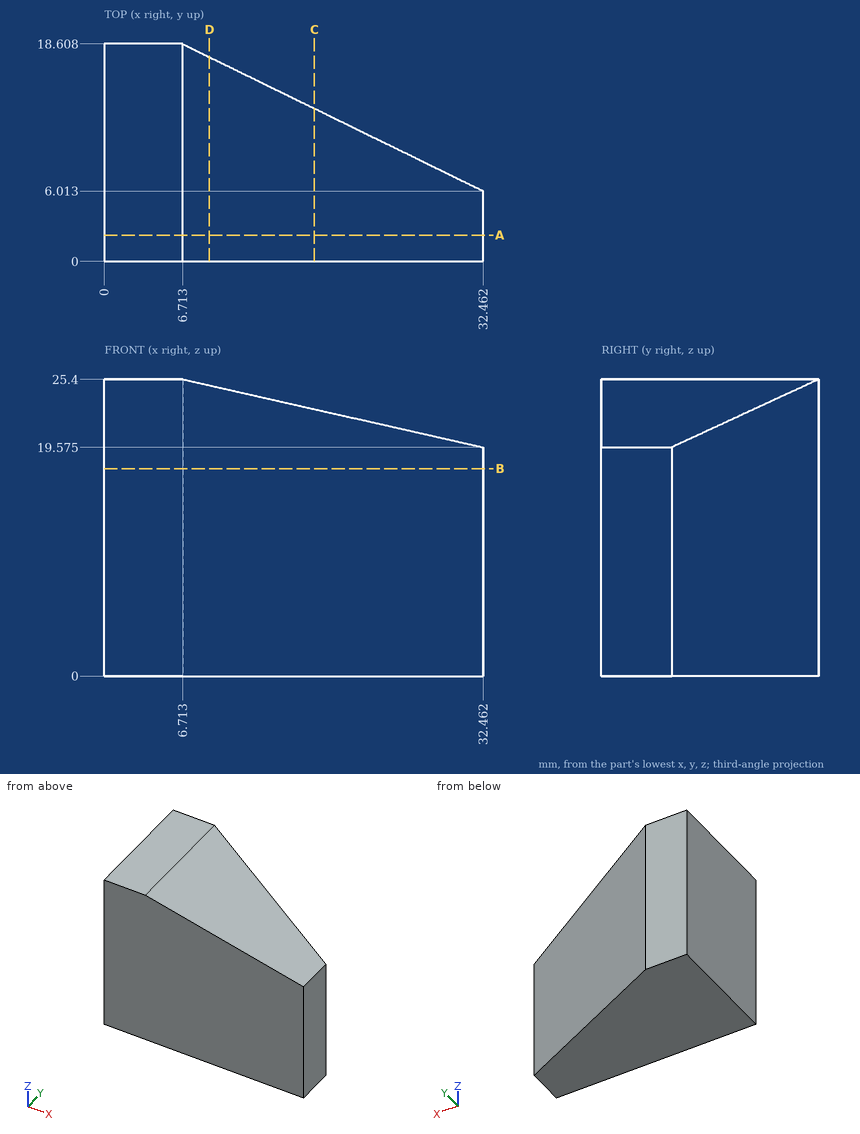
Verification items for this drawing (mm, ordinates from the low corner). Round coordinates to 2 decimals unless told otherwise and drop trailing zeros. Order: outer loops, then holes, each group sorted by start corner. A loop starts at its lowest first (then second) coordinate and runs counter-clockwise, first axis right, second up. Notation, with made-up numbers: (1.25, 64) - (16.25, 64) arc R19 cw to (16.25, 84) - close; hole circle Ø6 at (-34.5, -31.5). An arc over 180 degrees is marked (long way). Answer as CSV lines item,"result". Start each with the question number.
1) Section check D-D (x = 9). Record the cut outline in (y, z).
2) Scan lines: probe 1 along X at (y, z) = (14.25, 4.5) (1 decimal); probe 2 along Z at (x, y) = (24.5, 8.75) (1 decimal); probe 3 along Z at (x, y) = (15, 14.25) (1 decimal). Record each from-to range of solid material in increasing order.
3) Section check C-C (x = 18). Record the cut outline in (y, z).
4) Depth check by flat-ended pin: pin 1 (2 mm diameter, centred on x = 29, y = 11, fed in from +Z); pin 2 (6 mm diameter, centred on x = 25.5, z = 10, fed in from +Y) (1 decimal); pin 3 (5 mm diameter, centred on x = 27, z = 9.5, fed in from +Y). Enter the tip coordinate at first touch or a pass-through.
5) Section check A-A (y = 2.25). Record the cut outline in (x, z) (1 decimal).
6) Section check B-B (z = 17.75). Record the cut outline in (x, y).
Determined:
1,outline,"(0, 0) - (17.49, 0) - (17.49, 24.88) - (0, 24.88) - close"
2,probe 1,"0 to 15.6"
2,probe 2,"0 to 21.4"
2,probe 3,"0 to 23.5"
3,outline,"(0, 0) - (13.09, 0) - (13.09, 22.85) - (0, 22.85) - close"
4,pin 1,"through"
4,pin 2,"y = 10.9"
4,pin 3,"y = 9.91"
5,outline,"(0, 0) - (32.5, 0) - (32.5, 19.6) - (6.7, 25.4) - (0, 25.4) - close"
6,outline,"(0, 0) - (32.46, 0) - (32.46, 6.01) - (6.71, 18.61) - (0, 18.61) - close"
